Can you work these out from the drawing? Everything is in mm from the part's minimum corner. A direction names the side the tool comes from. Round coordinates to 2 decimals unless told otherwise and drop trailing zeros. Loops run counter-clockwise (first coordinate to the right, second up) from the corner with the lowest first, then second, coordinate; pieces in that order, holes last. Notation, with made-up numbers: (58, 19) - (72, 19) arc R37 cw to (72, 58) - close; hole circle Ø8 at (0.5, 69). An arc over 180 degrees is marked (long way). Answer as CSV lines item,"result". Start each with the question number.
1) Which directions (+Z, -Z, +X, -X, +Y, -Y) give clear straight access to the entire face, cutting with the end or side of a thin tool? Please do the marked faces 1 and 2.
2) Please list where these lines run through material, in increasing order: line 1 along Y through (x, z) = (31.75, 11.65); line 2 along Y through (x, z) = (31.75, 12.8) (1 decimal); line 3 along Y through (x, z) = (31.75, 5.5).
3) Suppose I cut it at C-C, the plane x = 26. Write out the boundary of the cut face in (y, z) (1 decimal).
4) Suppose I cut it at B-B, the plane z = 13.5. Count the separate pieces of the cut face and the enclosed holes in it, then the cut area to 3 significant figures.
5) I'm going to push flat-ended pins straight in: pin 1 Ø4 at (y, z) = (52, 6.5) entering from +X; pin 2 Ø5 at (x, z) = (22.5, 9) entering from +Y (1 decimal); pin 3 Ø2 at (x, y) = (22.5, 53) entering from -Z; pin 4 Ø10 at (x, y) = (53.75, 44.45) entering from +Z (1 decimal). Where does each tip first touch, or does it pass through?
6) Suppose I cut it at A-A, the plane y = 31.75. Write out the boundary of the cut face in (x, z) (1 decimal), then the cut area to 3 significant figures.
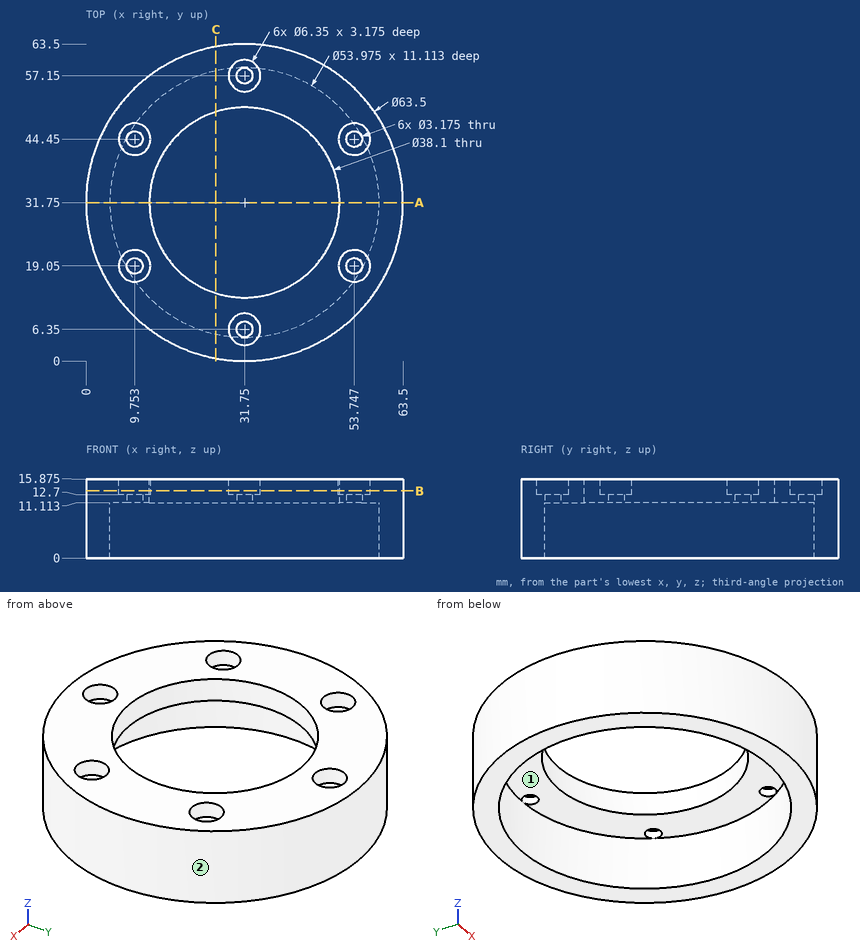
Filled sheet:
1,face 1,"-Z"
1,face 2,"+Z, -Z"
2,line 1,"0 to 4.76, 7.94 to 12.7, 50.8 to 55.56, 58.74 to 63.5"
2,line 2,"0 to 3.2, 9.5 to 12.7, 50.8 to 54, 60.3 to 63.5"
2,line 3,"0 to 4.76, 58.74 to 63.5"
3,outline,"(0.5, 0) - (5.4, 0) - (5.4, 11.1) - (13.6, 11.1) - (13.6, 15.9) - (0.5, 15.9) - close; (49.9, 11.1) - (58.1, 11.1) - (58.1, 0) - (63, 0) - (63, 15.9) - (49.9, 15.9) - close"
4,separate pieces,"1"
4,enclosed holes,"7"
4,area,"1,840 mm²"
5,pin 1,"x = 57.73"
5,pin 2,"y = 62.8"
5,pin 3,"z = 11.11"
5,pin 4,"z = 15.9"
6,outline,"(0, 0) - (4.8, 0) - (4.8, 11.1) - (12.7, 11.1) - (12.7, 15.9) - (0, 15.9) - close; (50.8, 11.1) - (58.7, 11.1) - (58.7, 0) - (63.5, 0) - (63.5, 15.9) - (50.8, 15.9) - close"
6,area,"227 mm²"
